Can you work these out from the model? Positions are in its coordinate system, mm. Face numbers are marked on the shaded views. Round coordinates to 2 decimals unless told otherwise and drop trailing zeros. Order: outer loops, then holes, each group sorted by start corner. A loop starts at its lowest first (then second) coordinate and runs counter-clockwise, first axis right, second up.
Q1. If we section it at D-D (x = -150): Please give me the cut outline in (y, z).
Q2. If we section it at B-B (z = 0): Please give me the cut outline in (x, y), plus the area to 3 significant figures.
Q3. If I drill on line 1 (Z direction, x = 150, y = 5.5); line 2 (X direction, y = 12.75, z = 0); line 3 (X direction, y = 3.5, z = 0), over which ranges is the centre line in solid material (lowest first)?
Q4. Will these pins go through, and if not, where does the flat tip stop? P1, Ø8, axis at y = 12, z = -48.5, coming from the +X side; P2, Ø10, axis at x = -136.5, y = 3, coming from the -Z side; P3, Ø1.5, axis at y = 2.5, z = -5.5, coming from the +X side.
Q5. If we section it at A-A (x = 0): Please give me the cut outline in (y, z).
Q6. If we section it at C-C (y = 6.75): Please give me the cut outline in (x, z).
Q7. We'd pull the mould along X, two halves only. Please class the marked faces 1 and 2: pulls with the +X half, pulls with the -X half, needs draft (parallel to the pull), parting line crosses it, or undercut.
from build123d import *

# Parameters (mm, degrees)
ESQUISSE1_R             = 50
BOSS_EXTRU_1_DEPTH      = 20
ESQUISSE2_R             = 67.8
ENL_V_MAT_EXTRU_1_DEPTH = 10


with BuildPart() as part:
    # Esquisse1 → Boss.-Extru.1 (new body)
    with BuildSketch(Plane(origin=(0, 0, 0), x_dir=(1, 0, 0), z_dir=(0, 1, 0))):
        with BuildLine():
            Line((172.912878475, 10), (188.729833462, 10))
            ThreePointArc((188.729833462, 10), (167.293491098, 36.068478837), (133.545454545, 36.458852613))
            ThreePointArc((133.545454545, 36.458852613), (91.415195679, 31.543703023), (54.181034483, 51.859574838))
            ThreePointArc((54.181034483, 51.859574838), (0, 75), (-54.181034483, 51.859574838))
            ThreePointArc((-54.181034483, 51.859574838), (-91.415195679, 31.543703023), (-133.545454545, 36.458852613))
            ThreePointArc((-133.545454545, 36.458852613), (-167.293491098, 36.068478837), (-188.729833462, 10))
            Line((-188.729833462, 10), (-172.912878475, 10))
            ThreePointArc((-172.912878475, 10), (-125, 0), (-172.912878475, -10))
            Line((-172.912878475, -10), (-188.729833462, -10))
            ThreePointArc((-188.729833462, -10), (-167.293491098, -36.068478837), (-133.545454545, -36.458852613))
            ThreePointArc((-133.545454545, -36.458852613), (-91.415195679, -31.543703023), (-54.181034483, -51.859574838))
            ThreePointArc((-54.181034483, -51.859574838), (0, -75), (54.181034483, -51.859574838))
            ThreePointArc((54.181034483, -51.859574838), (91.415195679, -31.543703023), (133.545454545, -36.458852613))
            ThreePointArc((133.545454545, -36.458852613), (167.293491098, -36.068478837), (188.729833462, -10))
            Line((188.729833462, -10), (172.912878475, -10))
            ThreePointArc((172.912878475, -10), (125, 0), (172.912878475, 10))
        make_face()
        with Locations(Location((0, 0, 0), (0, 0, 270))):
            Circle(ESQUISSE1_R, mode=Mode.SUBTRACT)
    extrude(amount=BOSS_EXTRU_1_DEPTH)

    # Esquisse2 → Enlèv. mat.-Extru.1 (cut)
    with BuildSketch(Plane(origin=(0, 20, 0), x_dir=(1, 0, 0), z_dir=(0, 1, 0))):
        with Locations(Location((0, 0, 0), (0, 0, 270))):
            Circle(ESQUISSE2_R)
    extrude(amount=-ENL_V_MAT_EXTRU_1_DEPTH, mode=Mode.SUBTRACT)


solid = part.part
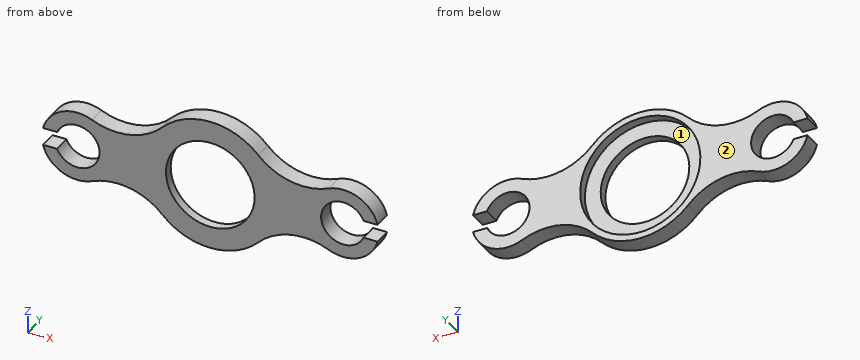
Solution:
1. outline: (0, -40) - (20, -40) - (20, -25) - (0, -25) - close; (0, 25) - (20, 25) - (20, 40) - (0, 40) - close
2. outline: (-125, 0) - (-50, 0) - (-50, 10) - (-67.8, 10) - (-67.8, 20) - (-125, 20) - close; (50, 0) - (125, 0) - (125, 20) - (67.8, 20) - (67.8, 10) - (50, 10) - close
2. area: 2,640 mm2
3. line 1: z = -40 to -25, 25 to 40
3. line 2: x = -125 to -67.8, 67.8 to 125
3. line 3: x = -125 to -50, 50 to 125
4. P1: stops at x = 62.43
4. P2: stops at z = -39.09
4. P3: stops at x = 125.79
5. outline: (0, -75) - (20, -75) - (20, -67.8) - (10, -67.8) - (10, -50) - (0, -50) - close; (0, 50) - (10, 50) - (10, 67.8) - (20, 67.8) - (20, 75) - (0, 75) - close
6. outline: (-188.73, -10) arc R40 ccw to (-133.55, -36.46) arc R70 cw to (-54.18, -51.86) arc R75 ccw to (54.18, -51.86) arc R70 cw to (133.55, -36.46) arc R40 ccw to (188.73, -10) - (172.91, -10) arc R25 cw (long way) to (172.91, 10) - (188.73, 10) arc R40 ccw to (133.55, 36.46) arc R70 cw to (54.18, 51.86) arc R75 ccw to (-54.18, 51.86) arc R70 cw to (-133.55, 36.46) arc R40 ccw to (-188.73, 10) - (-172.91, 10) arc R25 cw (long way) to (-172.91, -10) - close; hole circle Ø100 at (0, 0)
7. face 1: undercut
7. face 2: needs draft
